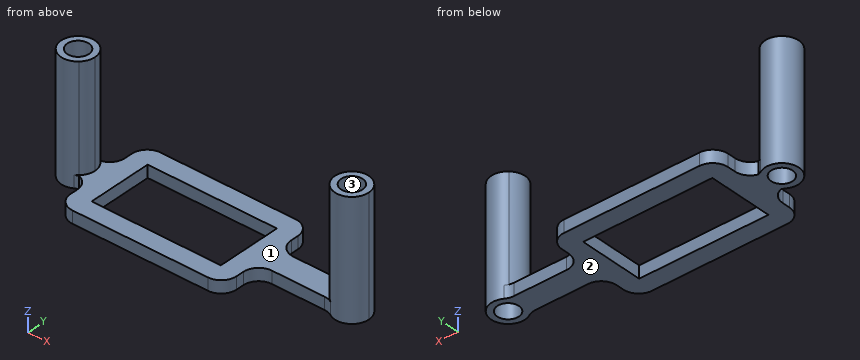
```python
from build123d import *

# Parameters (mm, degrees)
F1_DEPTH    = 4
F0_R        = 3.5
F2_DEPTH    = 38
F0_W        = 6
F0_H        = 8
F3_DEPTH    = 4
F4_T1_DEPTH = 4
F4_T3_DEPTH = 29


# Not quite as in the source:
# - a fillet or chamfer that OpenCascade refuses, or shapes differently, is made with other operations: its cross-section is extruded or revolved along the edge and cut away or added


with BuildPart() as f1:
    # F0 (on Top) → F1 (new body)
    with BuildSketch(Plane.XY):
        with BuildLine():
            ThreePointArc((-40.7250827824, 4), (-39.4496512647, 2.1780674121), (-39, 0))
            ThreePointArc((-39, 0), (-39.4496512647, -2.1780674121), (-40.7250827824, -4))
            Line((-40.7250827824, -4), (-37, -4))
            Line((-37, -4), (-37, 4))
            Line((-37, 4), (-40.7250827824, 4))
        make_face()
    extrude(amount=F1_DEPTH)

    # F0 (on Top) → F2 (join)
    with BuildSketch(Plane.XY):
        with BuildLine():
            ThreePointArc((-40.7250827824, -4), (-39.4496512647, -2.1780674121), (-39, 0))
            ThreePointArc((-39, 0), (-39.4496512647, 2.1780674121), (-40.7250827824, 4))
            ThreePointArc((-40.7250827824, 4), (-50, 0), (-40.7250827824, -4))
        make_face()
        with Locations((-44.5, 0)):
            Circle(F0_R, mode=Mode.SUBTRACT)
    extrude(amount=F2_DEPTH)



with BuildPart() as f1b:
    # F0 (on Top) → F1, piece 2 (new body)
    with BuildSketch(Plane.XY):
        with BuildLine():
            Line((40.7250827824, 4), (17, 4))
            Line((17, 4), (17, -4))
            Line((17, -4), (40.7250827824, -4))
            ThreePointArc((40.7250827824, -4), (39, 0), (40.7250827824, 4))
        make_face()
    extrude(amount=F1_DEPTH)

    # F0 (on Top) → F2, piece 2 (join)
    with BuildSketch(Plane.XY):
        with BuildLine():
            ThreePointArc((50, 0), (46.6780674121, 5.0503487353), (40.7250827824, 4))
            ThreePointArc((40.7250827824, 4), (39, 0), (40.7250827824, -4))
            ThreePointArc((40.7250827824, -4), (46.6780674121, -5.0503487353), (50, 0))
        make_face()
        with Locations((44.5, 0)):
            Circle(F0_R, mode=Mode.SUBTRACT)
    extrude(amount=F2_DEPTH)


with BuildPart() as f1_1:
    add(f1.part)

    add(f1b.part)  # F3 merges F1b
    # F0 (on Top) → F3 (join)
    with BuildSketch(Plane.XY):
        Polygon((-31, -4), (-37, -4), (-37, -16.5), (17, -16.5), (17, -4), (11, -4), (11, -10.5), (-31, -10.5), align=None)
        Polygon((-37, 16.5), (-37, 4), (-31, 4), (-31, 10.5), (11, 10.5), (11, 4), (17, 4), (17, 16.5), align=None)
        with Locations((-34, 0)):
            Rectangle(F0_W, F0_H)
        with Locations((14, 0)):
            Rectangle(F0_W, F0_H)
    extrude(amount=F3_DEPTH)

    # F4: fillet of radius 5 on 12 edges, made by hand

    # F4_s2 → F4_t1 (join)
    with BuildSketch(Plane.XY):
        with BuildLine():
            ThreePointArc((-39.0916730868, 4), (-40.4279792964, 4.1818794417), (-41.667066855, 4.7142857143))
            ThreePointArc((-41.667066855, 4.7142857143), (-41.1768279274, 4.3825252282), (-40.7250827824, 4))
            Line((-40.7250827824, 4), (-39.0916730868, 4))
        make_face()
        with BuildLine():
            ThreePointArc((-37, 9), (-38.4644660941, 5.4644660941), (-42, 4))
            Line((-42, 4), (-37, 4))
            Line((-37, 4), (-37, 9))
        make_face()
        with BuildLine():
            ThreePointArc((-37, -9), (-38.4644660941, -5.4644660941), (-42, -4))
            Line((-42, -4), (-37, -4))
            Line((-37, -4), (-37, -9))
        make_face()
        with BuildLine():
            ThreePointArc((-39.0916730868, -4), (-40.4279792964, -4.1818794417), (-41.667066855, -4.7142857143))
            ThreePointArc((-41.667066855, -4.7142857143), (-41.1768279274, -4.3825252282), (-40.7250827824, -4))
            Line((-40.7250827824, -4), (-39.0916730868, -4))
        make_face()
        with BuildLine():
            ThreePointArc((17, 9), (18.4644660941, 5.4644660941), (22, 4))
            Line((22, 4), (17, 4))
            Line((17, 4), (17, 9))
        make_face()
        with BuildLine():
            ThreePointArc((17, -9), (18.4644660941, -5.4644660941), (22, -4))
            Line((22, -4), (17, -4))
            Line((17, -4), (17, -9))
        make_face()
        with BuildLine():
            ThreePointArc((39.0916730868, -4), (40.4279792964, -4.1818794417), (41.667066855, -4.7142857143))
            ThreePointArc((41.667066855, -4.7142857143), (41.1768279274, -4.3825252282), (40.7250827824, -4))
            Line((40.7250827824, -4), (39.0916730868, -4))
        make_face()
        with BuildLine():
            ThreePointArc((41.667066855, 4.7142857143), (40.4279792964, 4.1818794417), (39.0916730868, 4))
            Line((39.0916730868, 4), (40.7250827824, 4))
            ThreePointArc((40.7250827824, 4), (41.1768279274, 4.3825252282), (41.667066855, 4.7142857143))
        make_face()
    extrude(amount=F4_T1_DEPTH)

    # F4_s4 → F4_t3 (cut)
    with BuildSketch(Plane.XY.offset(-12.5)):
        with BuildLine():
            ThreePointArc((12, 16.5), (15.5355339059, 15.0355339059), (17, 11.5))
            Line((17, 11.5), (17, 16.5))
            Line((17, 16.5), (12, 16.5))
        make_face()
        with BuildLine():
            ThreePointArc((-37, 11.5), (-35.5355339059, 15.0355339059), (-32, 16.5))
            Line((-32, 16.5), (-37, 16.5))
            Line((-37, 16.5), (-37, 11.5))
        make_face()
        with BuildLine():
            ThreePointArc((-32, -16.5), (-35.5355339059, -15.0355339059), (-37, -11.5))
            Line((-37, -11.5), (-37, -16.5))
            Line((-37, -16.5), (-32, -16.5))
        make_face()
        with BuildLine():
            ThreePointArc((12, -16.5), (15.5355339059, -15.0355339059), (17, -11.5))
            Line((17, -11.5), (17, -16.5))
            Line((17, -16.5), (12, -16.5))
        make_face()
    extrude(amount=F4_T3_DEPTH, mode=Mode.SUBTRACT)


solid = f1_1.part
```
Part model, mm, in its own coordinate system. Face numbers are marked on the shaded views. Coordinates: 2 decimals unless noted, no trailing zeros. Order: outer loops, then holes, each group sorted by start corner. A loop starts at its lowest first (then second) coordinate and runs counter-clockwise, first axis right, second up. Notation, with made-up numbers: (82.5, 58.25) -> (123.5, 58.25) arc R16 ccw to (123.5, 77.25) -> close; hole circle Ø7 at (-29, -10.75). An arc over 180 degrees is marked (long way). Put each result on its own line as item: value. Start each with the question number.
(1) Pin check, flat tips, straight feed: pin 1 Ø1 at (x, z) = (39.5, 12) entering from -Y; pin 2 Ø0.8 at (y, z) = (-10, 2) entering from -X; pin 3 Ø3 at (x, z) = (29, 2.5) entering from +Y. Stop position of each tip, or through.
(2) Band-saw the part on D-D (y = 8). Give the cut face in (x, z), then the cut area to 3 significant figures.
(3) Band-saw the part on C-C (y = -2.5). Give the cut face in (x, z), then the cut area to 3 significant figures.
(4) Band-saw the part on A-A (z = 32). Give the cut face in (x, y).
(5) Probe line 1 along Y through (x, z) = (44.5, 29.5); line 2 along X through (y, z) = (-1, 15); line 3 along Z through (x, y) = (-35, -15). List the from-to ranges inside material, lowest first. Write a range as [from, to].
(6) Mould opens along X. For the marked faces 1, 2 and 3 say: pulls with the +X half, pulls with the -X half, needs draft (parallel to the pull), parting line crosses it, or undercut.
(7) Band-saw the part on B-B (x = -44.5). Give the cut face in (y, z).
Determined:
1. pin 1: stops at y = -3.16
1. pin 2: stops at x = -37
1. pin 3: stops at y = 4
2. outline: (-37.1, 0) -> (-31, 0) -> (-31, 4) -> (-37.1, 4) -> close; (11, 0) -> (17.1, 0) -> (17.1, 4) -> (11, 4) -> close
2. area: 48.8 mm²
3. outline: (-49.4, 0) -> (-46.95, 0) -> (-46.95, 38) -> (-49.4, 38) -> close; (-42.05, 0) -> (-31, 0) -> (-31, 4) -> (-39.6, 4) -> (-39.6, 38) -> (-42.05, 38) -> close; (11, 0) -> (42.05, 0) -> (42.05, 38) -> (39.6, 38) -> (39.6, 4) -> (11, 4) -> close; (46.95, 0) -> (49.4, 0) -> (49.4, 38) -> (46.95, 38) -> close
3. area: 521 mm²
4. outline: circle Ø11 at (-44.5, 0); circle Ø11 at (44.5, 0); hole circle Ø7 at (-44.5, 0); hole circle Ø7 at (44.5, 0)
5. line 1: y = [-5.5, -3.5], [3.5, 5.5]
5. line 2: x = [-49.91, -47.85], [-41.15, -39.09], [39.09, 41.15], [47.85, 49.91]
5. line 3: z = [0, 4]
6. face 1: undercut
6. face 2: needs draft
6. face 3: undercut
7. outline: (-5.5, 0) -> (-3.5, 0) -> (-3.5, 38) -> (-5.5, 38) -> close; (3.5, 0) -> (5.5, 0) -> (5.5, 38) -> (3.5, 38) -> close
